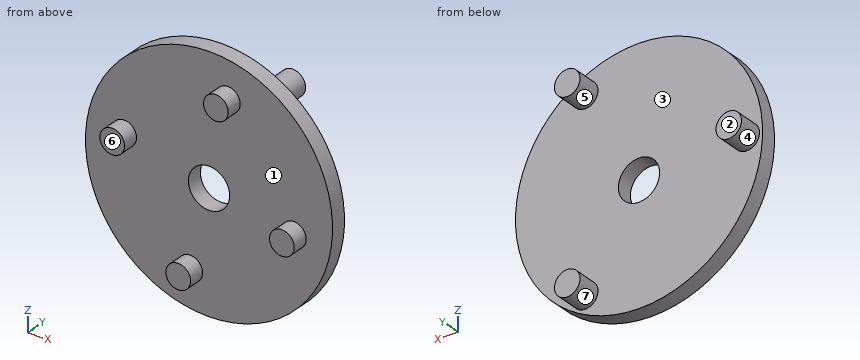
```python
from build123d import *

# Parameters (mm, degrees)
SKETCH1_R           = 150
SKETCH1_R_2         = 25
BOSS_EXTRUDE1_DEPTH = 20
SKETCH2_R           = 15.517679246
BOSS_EXTRUDE2_DEPTH = 30
SKETCH3_R           = 15.012096723
BOSS_EXTRUDE3_DEPTH = 20


with BuildPart() as part:
    # Sketch1 → Boss-Extrude1 (new body)
    with BuildSketch(Plane(origin=(0, 0, 0), x_dir=(1, 0, 0), z_dir=(0, 1, 0))):
        with Locations(Location((0, 0, 0), (0, 0, 270))):
            Circle(SKETCH1_R)
        with Locations(Location((0, 4.724194593, 0), (0, 0, 270))):
            Circle(SKETCH1_R_2, mode=Mode.SUBTRACT)
    extrude(amount=BOSS_EXTRUDE1_DEPTH)

    # Sketch2 → Boss-Extrude2 (add)
    with BuildSketch(Plane(origin=(0, 20, 0), x_dir=(1, 0, 0), z_dir=(0, 1, 0))):
        with Locations(Location((-130.753213973, 0, 0), (0, 0, 270))):
            Circle(SKETCH2_R)
        with Locations(Location((65.376606987, 113.235604927, 0), (0, 0, 270))):
            Circle(SKETCH2_R)
        with Locations(Location((65.376606987, -113.235604927, 0), (0, 0, 270))):
            Circle(SKETCH2_R)
    extrude(amount=BOSS_EXTRUDE2_DEPTH)

    # Sketch3 → Boss-Extrude3 (add)
    with BuildSketch(Plane.XZ):
        with Locations(Location((-103.00688249, 22.854430971, 0), (0, 0, 90))):
            Circle(SKETCH3_R)
        with Locations(Location((22.854430971, 103.00688249, 0), (0, 0, 90))):
            Circle(SKETCH3_R)
        with Locations(Location((103.00688249, -22.854430971, 0), (0, 0, 90))):
            Circle(SKETCH3_R)
        with Locations(Location((-22.854430971, -103.00688249, 0), (0, 0, 90))):
            Circle(SKETCH3_R)
    extrude(amount=BOSS_EXTRUDE3_DEPTH)


solid = part.part
```
Geometry check sheet. Reference: the model listing, model coordinates, mm. Face numbers are marked on the shaded views. A direction names the side the tool comes from. Round coordinates to 2 decimals unless told otherwise and drop trailing zeros. Loops run counter-clockwise (first coordinate to the right, second up) from the corner with the lowest first, then second, coordinate; pieces in that order, holes last. Notation, with made-up numbers: (19.25, 10.25) - (26.25, 10.25) arc R22 ccw to (26.25, 29.25) - close; hole circle Ø10 at (73, 13.5). An arc over 180 degrees is marked (long way). Write item = value, one per line. Start each with the question number.
1. Section check C-C on y = 29. Enter the section's corners in (x, z), then the cut area to 3 significant figures.
2. Thickness scan on line 1 (Y direction, x = 24.5, z = -108); line 2 (Y direction, x = -26, z = -115); line 3 (X direction, y = 33.5, z = -114). Record the ranges inside material, lowest first.
3. Section check A-A on z = 0. Enter the section's corners in (x, y), then the cut area to 3 significant figures.
4. Depth check by flat-ended pin: pin 1 (5 mm diameter, centred on x = 69.5, y = 4.5, fed in from -Z); pin 2 (10 mm diameter, centred on y = 3.5, z = -79.5, fed in from -X); pin 3 (2 mm diameter, centred on x = 97.5, y = 13, fed in from +Z). Enter the tip coordinate at first touch or a pass-through.
5. Set-up check for the marked faces 1, 2 and 3: record each of +Z, -Z, +X, -X, +Y, -Y from which the full face is reachable in a straight line by a thin tool's end or side.
6. Section check D-D on x = 60.5. Enter the section's corners in (y, z), then the cut area to 3 significant figures.
7. Mould release check, pull along Z, two halves, no side actions. Record for the marked faces 4, 5, 6 and 7: released by +Z, released by -Z, zero draft, split by the parting line, or undercut.
8. Section check B-B on x = 0. Enter the section's corners in (y, z).
Working result:
q1.outline = circle Ø31.04 at (-130.75, 0); circle Ø31.04 at (65.38, -113.24); circle Ø31.04 at (65.38, 113.24)
q1.area = 2,270 mm^2
q2.line_1 = 0 to 20
q2.line_2 = -20 to 20
q2.line_3 = 49.88 to 80.88
q3.outline = (-150, 0) - (-24.55, 0) - (-24.55, 20) - (-115.24, 20) - (-115.24, 50) - (-146.27, 50) - (-146.27, 20) - (-150, 20) - close; (24.55, 0) - (150, 0) - (150, 20) - (24.55, 20) - close
q3.area = 5,950 mm^2
q4.pin_1 = -134.21
q4.pin_2 = -130.19
q4.pin_3 = 114.84
q5.face_1 = -Y
q5.face_2 = +Z, -Z, +X, -X, +Y
q5.face_3 = +Y
q6.outline = (0, -137.26) - (20, -137.26) - (20, -127.97) - (50, -127.97) - (50, -98.5) - (20, -98.5) - (20, 98.5) - (50, 98.5) - (50, 127.97) - (20, 127.97) - (20, 137.26) - (0, 137.26) - close
q6.area = 7,260 mm^2
q7.face_4 = split by the parting line
q7.face_5 = undercut
q7.face_6 = zero draft
q7.face_7 = undercut
q8.outline = (0, -150) - (20, -150) - (20, -29.72) - (0, -29.72) - close; (0, 20.28) - (20, 20.28) - (20, 150) - (0, 150) - close
